Geometry check sheet. Reference: the model listing, model coordinates, mm. Face numbers are marked on the shaded views. Round coordinates to 2 decimals unless told otherwise and drop trailing zeros. Write each loop counter-clockwise with the first axis right and the second up, starting at its lowest first coordinate (ties: lowest second). Pieces come first, ordered by that corner, then holes. Notation, with made-up numbers: (24.5, -27) -> (78.5, -27) arc R35 cw to (78.5, 9) -> close; hole circle Ø1 at (32.5, 54.5). An arc over 180 degrees is marked (long way). Return JSON: item names as keys, results as strings. Group by question number.
from build123d import *

# Parameters (mm, degrees)
SKETCH_1_W               = 30
SKETCH_1_H               = 50
SKETCH_1_W_2             = 26
SKETCH_1_H_2             = 46
EXTRUDE_1_DEPTH          = 300
CUT_EXTRUDE_2_DEPTH      = 302.413337462
CUT_EXTRUDE_2_DEPTH_BACK = 302.413337462
SKETCH_3_R               = 1.95
CUT_EXTRUDE_3_DEPTH      = 8
CUT_EXTRUDE_4_DEPTH      = 13
SKETCH_6_W               = 25
SKETCH_6_H               = 2
SKETCH_6_W_2             = 10.885639634
CUT_EXTRUDE_5_DEPTH      = 5
SKETCH_7_W               = 25
SKETCH_7_H               = 2
CUT_EXTRUDE_6_DEPTH      = 10


with BuildPart() as part:
    # 스케치1 → 보스-돌출1 (new body)
    with BuildSketch(Plane.XY):
        Rectangle(SKETCH_1_W, SKETCH_1_H)
        Rectangle(SKETCH_1_W_2, SKETCH_1_H_2, mode=Mode.SUBTRACT)
    extrude(amount=EXTRUDE_1_DEPTH)

    # 스케치3 → 컷-돌출2 (cut, two sides: drawn at the far end of the back side and taken through both)
    with BuildSketch(Plane(origin=(0, 0, 0), x_dir=(0, 0, -1), z_dir=(1, 0, 0)).offset(-CUT_EXTRUDE_2_DEPTH_BACK)):
        with Locations((-85.2, 15)):
            Circle(SKETCH_3_R)
        with Locations((-24.5, 2)):
            Circle(SKETCH_3_R)
    extrude(amount=CUT_EXTRUDE_2_DEPTH + CUT_EXTRUDE_2_DEPTH_BACK, mode=Mode.SUBTRACT)

    # 스케치4 → 컷-돌출3 (cut, symmetric)
    with BuildSketch(Plane(origin=(0, 0, 0), x_dir=(0, 0, -1), z_dir=(1, 0, 0))):
        Polygon((-20, 25), (-20, -23), (-48, -23), (-74, -23), (-97.25, -23), (-97.25, 25), align=None)
    extrude(amount=CUT_EXTRUDE_3_DEPTH, both=True, mode=Mode.SUBTRACT)

    # 스케치5 → 컷-돌출4 (cut, symmetric)
    with BuildSketch(Plane(origin=(0, 0, 0), x_dir=(0, 0, -1), z_dir=(1, 0, 0))):
        Polygon((-92, 23), (-92, 25), (-200, 25), (-200, -25), (-92, -25), align=None)
    extrude(amount=CUT_EXTRUDE_4_DEPTH, both=True, mode=Mode.SUBTRACT)

    # 스케치6 → 컷-돌출5 (cut, symmetric)
    with BuildSketch(Plane(origin=(0, 0, 0), x_dir=(0, 0, -1), z_dir=(1, 0, 0))):
        with Locations((-52.975965068, -24)):
            Rectangle(SKETCH_6_W, SKETCH_6_H)
        with Locations((-83.750343722, -24)):
            Rectangle(SKETCH_6_W_2, SKETCH_6_H)
    extrude(amount=CUT_EXTRUDE_5_DEPTH, both=True, mode=Mode.SUBTRACT)

    # 스케치7 → 컷-돌출6 (cut, symmetric)
    with BuildSketch(Plane(origin=(0, 0, 0), x_dir=(0, 0, -1), z_dir=(1, 0, 0))):
        with Locations((-12.5, -24)):
            Rectangle(SKETCH_7_W, SKETCH_7_H)
    extrude(amount=CUT_EXTRUDE_6_DEPTH, both=True, mode=Mode.SUBTRACT)


solid = part.part
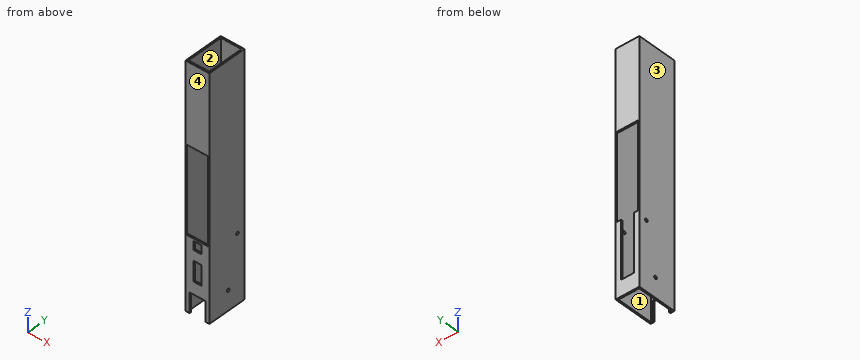
1) Sectioned sample at C-C on y = -15.5. Enter the section's corners in (x, z), and give its area (3 significant figures).
2) Sectioned sample at A-A on x = 1. Enter the section's corners in (y, z), and give its area (3 significant figures).
3) Material ranges on probe 1 along Y at (x, z) = (2, 214); probe 2 along X at (y, z) = (-20, 284); probe 3 along Z at (x, y) = (-14.05, 15), recorded low to high. Write a range as [from, to].
4) Sectioned sample at D-D on z = 225.5. Enter the section's corners in (x, y).
5) Sectioned sample at B-B on z = 167. Enter the section's corners in (x, y), and give its area (3 significant figures).
6) Mould release check, pull along Y, two halves, no side actions. Record for the marked faces 1, 2, 3 and 4: +Y half, -Y half, draft (parallel to the pull), parting line (faces both ways), or undercut.
7) Go/stop test with flat-tipped pins: P1, Ø2, axis at x = 2, y = -24, coming from the -Z side; P2, Ø8, axis at x = 10.5, y = 8.5, coming from the -Z side; P3, Ø3.5, axis at y = 2, z = 24.5, coming from the -X side. Record where each tip stops, or that it passes through.
Evaluation:
{
 "1": {"outline": "(-15, 0) -> (-13, 0) -> (-13, 300) -> (-15, 300) -> close; (13, 0) -> (15, 0) -> (15, 300) -> (13, 300) -> close", "area": "1,200 mm2"},
 "2": {"outline": "(-25, 25) -> (-23, 25) -> (-23, 40.48) -> (-25, 40.48) -> close; (-25, 65.48) -> (-23, 65.48) -> (-23, 78.31) -> (-25, 78.31) -> close; (-25, 89.19) -> (-23, 89.19) -> (-23, 92) -> (-25, 92) -> close; (-25, 200) -> (-23, 200) -> (-23, 300) -> (-25, 300) -> close; (23, 0) -> (25, 0) -> (25, 20) -> (23, 20) -> close; (23, 200) -> (25, 200) -> (25, 300) -> (23, 300) -> close", "area": "502 mm2"},
 "3": {"probe 1": "y = [-25, -23], [23, 25]", "probe 2": "x = [-15, -13], [13, 15]", "probe 3": "z = [0, 83.25], [87.15, 300]"},
 "4": {"outline": "(-15, -25) -> (15, -25) -> (15, 25) -> (-15, 25) -> close; hole (-13, -23) -> (13, -23) -> (13, 23) -> (-13, 23) -> close"},
 "5": {"outline": "(-15, -25) -> (-13, -25) -> (-13, 25) -> (-15, 25) -> close; (13, -25) -> (15, -25) -> (15, 25) -> (13, 25) -> close", "area": "200 mm2"},
 "6": {"face 1": "undercut", "face 2": "undercut", "face 3": "draft", "face 4": "-Y half"},
 "7": {"P1": "stops at z = 25", "P2": "stops at z = 0", "P3": "passes through"}
}
